Design review of the part shown in the three views and the two pictorial views. Dimensions are in mm from the part's minimum x, y and z. Round coordinates to 2 decimals unless told otherwise and drop trailing zeros. Loops run counter-clockwise (first coordinate to the right, second up) from the corner with the lowest first, then second, coordinate; pieces in that order, holes last. Notation, with made-up numbers: (67, -33) -> (82, -33) arc R30 ccw to (82, -8) -> close; hole circle Ø4 at (-37, 20.5). An arc over 180 degrees is marked (long way). One line per question, with ' | ' between items. Start each with the question number.
1. For pin 1 Ø1 at (x, y) = (64, 1) entering from -Z; pin 2 Ø1.3 at (y, z) = (2, 47) entering from -X; pin 3 Ø0.8 at (x, y) = (128, 0.5) entering from +Z, all flat-tipped, find the tip position at first contact; note any pin that passes through.
2. Wall thickness on line 1 along X through (y, z) = (2.3, 12.5); line 2 along Z through (x, y) = (131, 1.8): over which ranges is each line inside the solid? List them lowest first.
3. Consider section A-A (z = 30.5). Write out the cut boundary in (x, y).
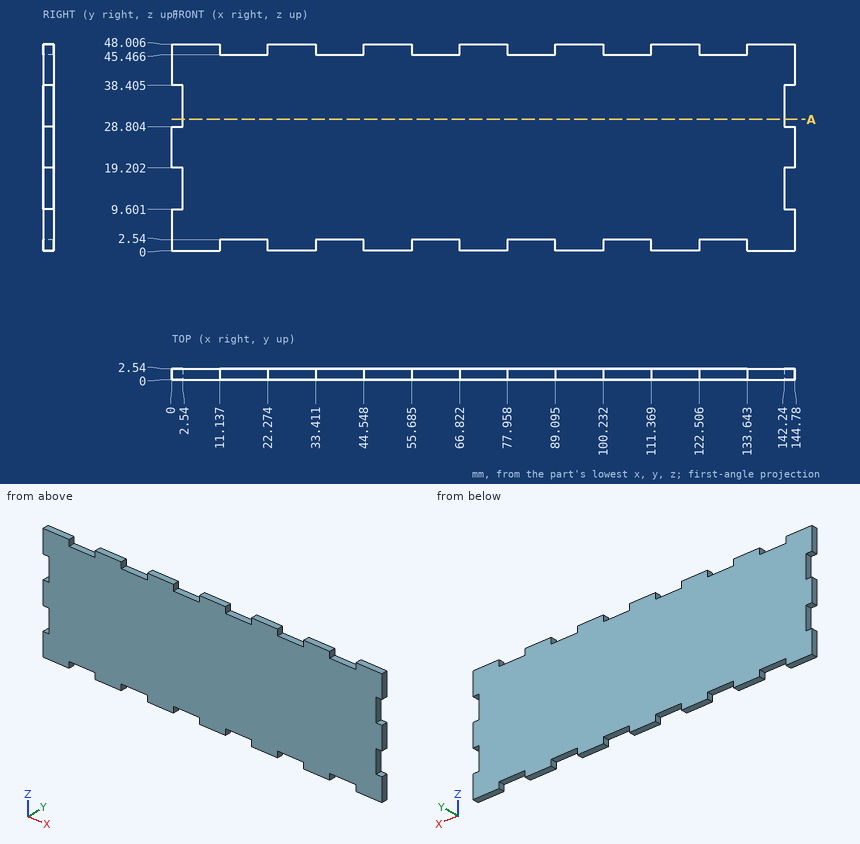
Answer block:
1) pin 1: stops at z = 2.54 | pin 2: stops at x = 0 | pin 3: stops at z = 45.47
2) line 1: x = 2.54 to 142.24 | line 2: z = 2.54 to 45.47
3) outline: (2.54, 0) -> (142.24, 0) -> (142.24, 2.54) -> (2.54, 2.54) -> close
